from build123d import *


with BuildPart() as part:
    # Sketch1 → Revolve1 (revolve)
    with BuildSketch(Plane.XY):
        Polygon((0, 0), (0, 24.80945), (0.762, 25.57145), (5.8166, 25.57145), (6.8707, 24.51735), (7.9248, 24.51735), (7.9248, 26.48585), (19.1008, 26.48585), (20.6248, 24.96185), (20.6248, 0), align=None)
    revolve(axis=Axis((20.6248, 0, 0), (-1, 0, 0)))

    # Sketch2 → Revolve2 (revolve)
    with BuildSketch(Plane.XY):
        with BuildLine():
            Line((6.477090712, 26.401681804), (7.789783697, 25.088988819))
            ThreePointArc((7.789783697, 25.088988819), (7.826981136, 24.999186258), (7.789783697, 24.909383697))
            Line((7.789783697, 24.909383697), (7.39775, 24.51735))
            Line((7.39775, 24.51735), (6.8707, 24.51735))
            Line((6.8707, 24.51735), (6.8707, 24.26335))
            Line((6.8707, 24.26335), (7.9248, 24.26335))
            Line((7.9248, 24.26335), (7.9248, 25.241340712))
            Line((7.9248, 25.241340712), (6.680290712, 26.48585))
            Line((6.680290712, 26.48585), (6.477090712, 26.48585))
            Line((6.477090712, 26.48585), (6.477090712, 26.401681804))
        make_face()
    revolve(axis=Axis((7.9248, 0, 0), (-1, 0, 0)))

    # Sketch3 → Cut-Revolve1 (revolve, cut)
    with BuildSketch(Plane.XY):
        Polygon((0, 0), (0, 20.5994), (0.762, 19.8374), (3.175, 19.8374), (3.175, 16.59255), (3.937, 15.83055), (12.7, 15.83055), (12.7, 0), align=None)
    revolve(axis=Axis((12.7, 0, 0), (-1, 0, 0)), mode=Mode.SUBTRACT)


solid = part.part
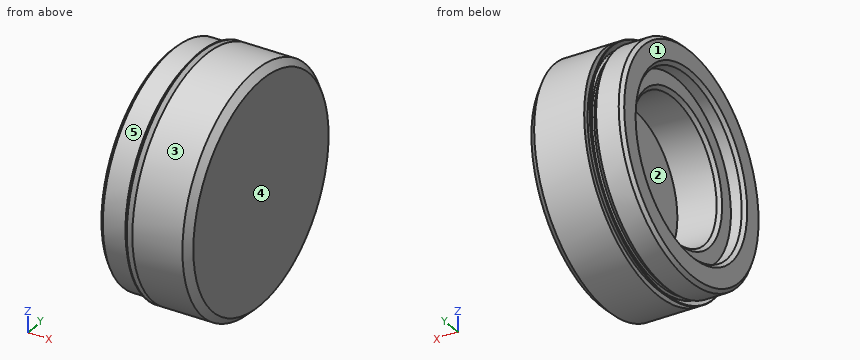
For this review, take the finished solid that the model builds, in its own axes (mm). Face numbers are marked on the shaded views. A direction names the side the tool comes from. Round coordinates to 2 decimals unless told otherwise and drop trailing zeros. Order: outer loops, then holes, each group sorted by start corner. A loop starts at its lowest first (then second) coordinate and runs counter-clockwise, first axis right, second up. Notation, with made-up numbers: M -18,50 L 26,50 A26 cw 26,71 Z; hole C 44,32.5 d6. An arc over 180 degrees is marked long. Use a Markdown table: item, result. Add a question column.
Item 1: To check wall thickness, follow line 1 along Z through (x, y) = (2.6, 0); line 2 along Y through (x, z) = (7, 0); line 3 along Y through (x, z) = (7.5, 21.5). State the ranges of each line that lie inside material, in increasing order.
Item 2: Add section B-B, the plane x = 17. Give the boundary of the cut face in (y, z).
Item 3: Tool access review of the marked faces 4 and 5: name each direction out of +Z, -Z, +X, -X, +Y, -Y from which nothing blocks a thin tool from reaching the whole face with its end or side.
Item 4: Mouldability with a two-part tool opening along Y and no side actions: class the marked faces 1, 2 and 3 as released by +Y, released by -Y, zero draft, split by the parting line, or undercut.
Item 5: Add section A-A, the plane x = 1.75. Give the boundary of the cut face in (y, z).
Item 6: Add section C-C, the plane x = 9.5. Give the boundary of the cut face in (y, z), then the cut area to 3 significant figures.
Item 7: Insertion check: pin 1 (5 mm diameter, centred on x = 4, z = -19, fed in from -Y); pin 2 (5 mm diameter, centred on x = 12.5, z = 9.5, fed in from +Y); pin 3 (3 mm diameter, centred on x = 6, y = 7.5, fed in from +Z). Each pin has a flat end and moves straight along its axis. Give the tip position at first contact, or say it passes through.
Geometry results:
| question | item | result |
|---|---|---|
| 1 | line 1 | z = -25.57 to -19.84, 19.84 to 25.57 |
| 1 | line 2 | y = -26.17 to -25.88, -24.52 to -15.83, 15.83 to 24.52, 25.88 to 26.17 |
| 1 | line 3 | y = -14.02 to -13.48, -11.99 to 11.99, 13.48 to 14.02 |
| 2 | outline | C 0,0 d52.97 |
| 3 | face 4 | +Z, -Z, +X, +Y, -Y |
| 3 | face 5 | -X |
| 4 | face 1 | zero draft |
| 4 | face 2 | undercut |
| 4 | face 3 | split by the parting line |
| 5 | outline | C 0,0 d51.14; hole C 0,0 d39.67 |
| 6 | outline | C 0,0 d52.97; hole C 0,0 d31.66 |
| 6 | area | 1,420 mm² |
| 7 | pin 1 | stops at y = -19.54 |
| 7 | pin 2 | stops at y = 25.54 |
| 7 | pin 3 | stops at z = 25.78 |
